Read the model definition and answer for the solid it produces. Units are mm, in the model's axes. Face numbers are marked on the shaded views. A direction names the side the tool comes from. Round coordinates to 2 decimals unless told otherwise and drop trailing zeros. Loops run counter-clockwise (first coordinate to the right, second up) from the corner with the lowest first, then second, coordinate; pieces in that order, holes last. Notation, with made-up numbers: (35.25, 84) -> (88.25, 84) arc R12 ccw to (88.25, 88) -> close; hole circle Ø7 at (-29, 35). An arc over 180 degrees is marked (long way). Put each result on its own line as item: value.
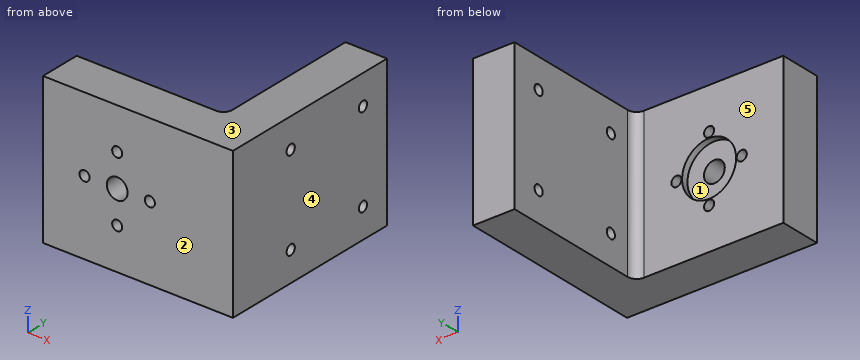
from build123d import *

# Parameters (mm, degrees)
BOSS_EXTRUDE1_DEPTH = 25
SKETCH3_R           = 3.5
CUT_EXTRUDE1_DEPTH  = 66.429351212
SKETCH4_R           = 1.7
CUT_EXTRUDE2_DEPTH  = 66.429351212
SKETCH5_R           = 1.7
CUT_EXTRUDE3_DEPTH  = 80.837334625
SKETCH6_R           = 9.1
CUT_EXTRUDE4_DEPTH  = 2.2
FILLET1_R           = 3


with BuildPart() as part:
    # Sketch2 → Boss-Extrude1 (new, symmetric)
    with BuildSketch(Plane.XY):
        Polygon((-34, 7), (16, 7), (16, 57), (30, 57), (30, 7), (30, -7), (-34, -7), align=None)
    extrude(amount=BOSS_EXTRUDE1_DEPTH, both=True)

    # Sketch3 → Cut-Extrude1 (cut, through all)
    with BuildSketch(Plane(origin=(0, 7, 0), x_dir=(1, 0, 0), z_dir=(0, 1, 0))):
        with Locations(Location((-9, 0, 0), (0, 0, 180))):
            Circle(SKETCH3_R)
    extrude(amount=-CUT_EXTRUDE1_DEPTH, mode=Mode.SUBTRACT)

    # Sketch4 → Cut-Extrude2 (cut, through all)
    with BuildSketch(Plane(origin=(0, 7, 0), x_dir=(1, 0, 0), z_dir=(0, 1, 0))):
        with Locations(Location((-9, 11, 0), (0, 0, 180))):
            Circle(SKETCH4_R)
        with Locations(Location((-20, 0, 0), (0, 0, 180))):
            Circle(SKETCH4_R)
        with Locations(Location((-9, -11, 0), (0, 0, 180))):
            Circle(SKETCH4_R)
        with Locations(Location((2, 0, 0), (0, 0, 180))):
            Circle(SKETCH4_R)
    extrude(amount=-CUT_EXTRUDE2_DEPTH, mode=Mode.SUBTRACT)

    # Sketch5 → Cut-Extrude3 (cut, through all)
    with BuildSketch(Plane.ZY.offset(-16)):
        with Locations((-15, 47)):
            Circle(SKETCH5_R)
        with Locations((-15, 17)):
            Circle(SKETCH5_R)
        with Locations((15, 17)):
            Circle(SKETCH5_R)
        with Locations((15, 47)):
            Circle(SKETCH5_R)
    extrude(amount=-CUT_EXTRUDE3_DEPTH, mode=Mode.SUBTRACT)

    # Sketch6 → Cut-Extrude4 (cut)
    with BuildSketch(Plane(origin=(0, 7, 0), x_dir=(1, 0, 0), z_dir=(0, 1, 0))):
        with Locations(Location((-9, 0, 0), (0, 0, 180))):
            Circle(SKETCH6_R)
    extrude(amount=-CUT_EXTRUDE4_DEPTH, mode=Mode.SUBTRACT)

    # Fillet1
    fillet1_edges = [part.edges().sort_by_distance(p)[0] for p in [
        (16, 7, 0),
    ]]
    fillet(fillet1_edges, radius=FILLET1_R)


solid = part.part
Item 1: The part is cut by section C-C (y = 2). Determine the outline of the cut face in (x, z), then the cut area to 3 significant figures.
Derived:
outline: (-34, -25) -> (30, -25) -> (30, 25) -> (-34, 25) -> close; hole circle Ø3.4 at (-20, 0); hole circle Ø7 at (-9, 0); hole circle Ø3.4 at (-9, -11); hole circle Ø3.4 at (-9, 11); hole circle Ø3.4 at (2, 0)
area: 3,130 mm^2
Item 2: For a pull along Z with two mould halves and no side action, classify the marked faces 1, 2 and 3 as pulls with the +Z half, pulls with the -Z half, needs draft (parallel to the pull), parting line crosses it, or undercut.
Derived:
face 1: undercut
face 2: needs draft
face 3: pulls with the +Z half
Item 3: The part is cut by section B-B (z = 11). Determine the outline of the cut face in (x, y), then the cut area to 3 significant figures.
Derived:
outline: (-34, -7) -> (-10.7, -7) -> (-10.7, 7) -> (-34, 7) -> close; (-7.3, -7) -> (30, -7) -> (30, 57) -> (16, 57) -> (16, 10) arc R3 cw to (13, 7) -> (-7.3, 7) -> close
area: 1,550 mm^2
Item 4: Find the intervals of material crossed by line 1 along Y through (x, z) = (20, -15); line 2 along Z through (x, y) = (2, 3.5); line 3 along X through (y, z) = (36.5, -5), in increasing order.
Derived:
line 1: y = -7 to 15.3, 18.7 to 45.3, 48.7 to 57
line 2: z = -25 to -1.7, 1.7 to 25
line 3: x = 16 to 30
Item 5: The part is cut by section A-A (x = -20). Determine the outline of the cut face in (y, z), then the cut area to 3 significant figures.
Derived:
outline: (-7, -25) -> (7, -25) -> (7, -1.7) -> (-7, -1.7) -> close; (-7, 1.7) -> (7, 1.7) -> (7, 25) -> (-7, 25) -> close
area: 652 mm^2
Item 6: The part is cut by section D-D (z = -15). Determine the outline of the cut face in (x, y).
Derived:
outline: (-34, -7) -> (30, -7) -> (30, 15.3) -> (16, 15.3) -> (16, 10) arc R3 cw to (13, 7) -> (-34, 7) -> close; (16, 18.7) -> (30, 18.7) -> (30, 45.3) -> (16, 45.3) -> close; (16, 48.7) -> (30, 48.7) -> (30, 57) -> (16, 57) -> close
Item 7: Flat-ended cylindrical pins translate along their axes: pin 1 Ø5 at (x, z) = (6.5, 16.5) entering from +Y; pin 2 Ø12 at (y, z) = (38, 1.5) entering from -X; pin 3 Ø5.5 at (x, z) = (-9, 0) entering from -Y; pin 4 Ø14.5 at (x, z) = (-9, 0) entering from +Y. Find the tip coordinate at first contact, or state that the pin passes through.
Derived:
pin 1: stops at y = 7
pin 2: stops at x = 16
pin 3: passes through
pin 4: stops at y = 4.8
Item 8: Which of the six approach directions +Z, -Z, +X, -X, +Y, -Y give full straight-line access (tool end or side, diameter ignored) to the marked faces 4 and 5?
Derived:
face 4: +Z, -Z, +X, +Y, -Y
face 5: +Z, -Z, -X, +Y
